Build history of the part. All positions in model axes, mm. Give positions to 0.01 mm unless a question says otherwise; leave off trailing zeros. Order: outer loops, then holes, each group sorted by start corner. A loop starts at its lowest first (then second) coordinate and runs counter-clockwise, first axis right, second up. Notation, with made-up numbers: (88, 78) - (143, 78) arc R21 ccw to (143, 100) - close; hole circle Ø9 at (71, -14). An arc over 180 degrees is marked (long way). Use a Markdown table: item, result. Add a question column.
(1) Flat gauge pin, fed straight in: pin 1 (1 mm diameter, centred on x = -43, y = 1, fed in from +Z). Where does the tip first touch, or does it go through?
(2) Slice it at A-A (z = -11.7). Write the cut outline in (x, y) (3 decimals).
(3) Slice it at C-C (x = -13). Write the cut outline in (y, z) (3 decimals), then the cut area to 3 significant figures.
(4) Slice it at B-B (y = 2). Write the cut outline in (x, z) (3 decimals), then the cut area to 3 significant figures.
(5) Wall check: line 1 (Z direction, x = -13, y = 2.1) (3 decimals); line 2 (X direction, y = 0.6, z = -13); line 3 (Z direction, x = -13.5, y = 2.8). Give the ranges that are in metal, low to high.
Autodesk Inventor part; units mm, degrees
ref_plane "YZ Plane" through (0, 0, 0) normal (1, 0, 0) x (0, 1, 0)
ref_plane "XZ Plane" through (0, 0, 0) normal (0, 1, 0) x (-1, 0, 0)
ref_plane "XY Plane" through (0, 0, 0) normal (0, 0, 1) x (1, 0, 0)
sketch "草图1" plane through (0, 0, 0) normal (0, 1, 0) x (-1, 0, 0)
  line L0 (0, 0) -> (53, 0)
  line L1 (53, 0) -> (53, -45)
  line L2 (53, -45) -> (0, -45)
  line L3 (0, -45) -> (0, 0)
  line L4 (53, -22.5) -> (49.1677, -22.5)
  line L5 (26.5, -45) -> (26.5, -38.7473)
  circle A0 centre (40, -33.3) radius 1.525
  circle A1 centre (40, -11.7) radius 1.525
  circle A2 centre (13, -33.3) radius 1.525
  circle A3 centre (13, -11.7) radius 1.525
  dimension "d0" = 45
  dimension "d1" = 53
  dimension "d2" = 10.8
  dimension "d3" = 13
  dimension "d4" = 3.05
extrude "拉伸1" add sketch "草图1" along normal blind 3
sketch "草图2" plane through (0, 3, 0) normal (0, 1, 0) x (1, 0, 0)
  line L0 (-52, 50.7806) -> (-1, 50.7806)
  line L1 (-1, 50.7806) -> (-1, -16.6208)
  line L2 (-1, -16.6208) -> (-52, -16.6208)
  line L3 (-52, -16.6208) -> (-52, 50.7806)
  line L4 (-53, 45) -> (-53, 0)
  line L5 (0, 0) -> (0, 45)
  line L6 (0, 0) -> (0, 45)
  line L7 (0, 45) -> (-53, 45)
  line L8 (-53, 45) -> (-53, 0)
  line L9 (-53, 0) -> (0, 0)
  circle A0 centre (-40, 33.3) radius 1.525
  circle A1 centre (-40, 11.7) radius 1.525
  circle A2 centre (-13, 33.3) radius 1.525
  circle A3 centre (-13, 11.7) radius 1.525
  point P0 (-1, 0)
  point P1 (-1, 45)
  point P2 (-52, 0)
  point P3 (-52, 45)
  dimension "d10" = 1
  dimension "d11" = 1
extrude "拉伸2" cut sketch "草图2" against normal blind 10 contours L3 L9 L4 L7 | L7 L5 L9 L1
chamfer "倒角2" distance 8 angle 45 4 edges at (-1, 1.5, 0) (-52, 1.5, 0) (-52, 1.5, -45) (-1, 1.5, -45)
sketch "草图3" plane through (0, 0, 0) normal (0, -1, 0) x (1, 0, 0)
  circle A0 centre (-40, -33.3) radius 1.525
  circle A1 centre (-13, -33.3) radius 1.525
  point P0 (0, 0)
  dimension "d17" = 27
properties part number "sh2"
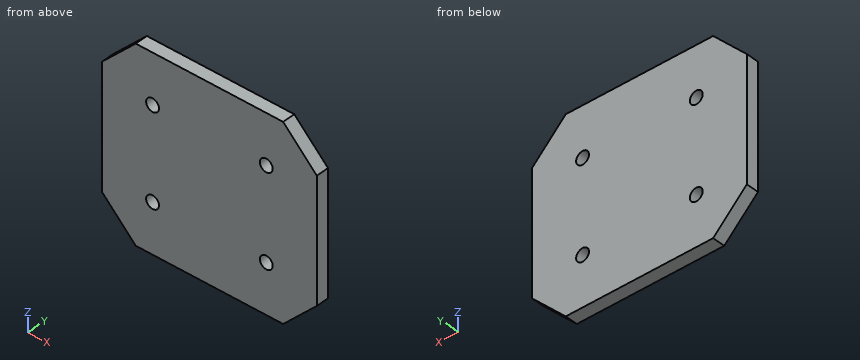
Solution:
| question | item | result |
|---|---|---|
| 1 | pin 1 | z = 0 |
| 2 | outline | (-52, 0) - (-41.525, 0) - (-41.525, 3) - (-52, 3) - close; (-38.475, 0) - (-14.525, 0) - (-14.525, 3) - (-38.475, 3) - close; (-11.475, 0) - (-1, 0) - (-1, 3) - (-11.475, 3) - close |
| 3 | outline | (0, -45) - (3, -45) - (3, -34.825) - (0, -34.825) - close; (0, -31.775) - (3, -31.775) - (3, -13.225) - (0, -13.225) - close; (0, -10.175) - (3, -10.175) - (3, 0) - (0, 0) - close |
| 3 | area | 117 mm2 |
| 4 | outline | (-52, -37) - (-44, -45) - (-9, -45) - (-1, -37) - (-1, -8) - (-9, 0) - (-44, 0) - (-52, -8) - close; hole circle Ø3.05 at (-40, -33.3); hole circle Ø3.05 at (-40, -11.7); hole circle Ø3.05 at (-13, -33.3); hole circle Ø3.05 at (-13, -11.7) |
| 4 | area | 2,140 mm2 |
| 5 | line 1 | -45 to -34.825, -31.775 to -13.225, -10.175 to 0 |
| 5 | line 2 | -52 to -40.8, -39.2 to -13.8, -12.2 to -1 |
| 5 | line 3 | -45 to -34.74, -31.86 to -13.14, -10.26 to 0 |
